from build123d import *

# Parameters (mm, degrees)
RESSALTO_EXTRUS_O1_DEPTH = 2
ESBO_O2_R                = 1.65
ESBO_O2_R_2              = 1.5
ESBO_O2_R_3              = 1
CORTE_EXTRUS_O1_DEPTH    = 3.0000001


with BuildPart() as part:
    # Esboço1 → Ressalto-extrusão1 (new body)
    with BuildSketch(Plane(origin=(0, 0, 0), x_dir=(1, 0, 0), z_dir=(0, 1, 0))):
        with BuildLine():
            Line((-57, 14.836150135), (-51, 9.5))
            Line((-51, 9.5), (-22.083647797, 9.5))
            add(Edge.make_bspline(
                [(22.083647797, 9.5), (0, 38), (-22.083647797, 9.5)],
                knots=[0.523598776, 0.523598776, 0.523598776, 2.617993878, 2.617993878, 2.617993878], degree=2, weights=[1, 0.5, 1]))
            Line((22.083647797, 9.5), (51, 9.5))
            Line((51, 9.5), (57, 14.836150135))
            Line((57, 14.836150135), (68, 14.836150135))
            Line((68, 14.836150135), (68, 8.836150135))
            Line((68, 8.836150135), (70.5, 8.836150135))
            Line((70.5, 8.836150135), (70.5, -7.163849865))
            Line((70.5, -7.163849865), (68, -7.163849865))
            Line((68, -7.163849865), (68, -13.163849865))
            Line((68, -13.163849865), (57, -13.163849865))
            Line((57, -13.163849865), (51, -9.5))
            Line((51, -9.5), (22.083647797, -9.5))
            add(Edge.make_bspline(
                [(-22.083647797, -9.5), (0, -38), (22.083647797, -9.5)],
                knots=[3.665191429, 3.665191429, 3.665191429, 5.759586532, 5.759586532, 5.759586532], degree=2, weights=[1, 0.5, 1]))
            Line((-22.083647797, -9.5), (-51, -9.5))
            Line((-51, -9.5), (-57, -13.163849865))
            Line((-57, -13.163849865), (-68, -13.163849865))
            Line((-68, -13.163849865), (-68, -7.163849865))
            Line((-68, -7.163849865), (-70.5, -7.163849865))
            Line((-70.5, -7.163849865), (-70.5, 8.836150135))
            Line((-70.5, 8.836150135), (-68, 8.836150135))
            Line((-68, 8.836150135), (-68, 14.836150135))
            Line((-68, 14.836150135), (-57, 14.836150135))
        make_face()
    extrude(amount=RESSALTO_EXTRUS_O1_DEPTH)

    # Esboço2 → Corte-extrusão1 (cut, through all)
    with BuildSketch(Plane(origin=(0, 2, 0), x_dir=(1, 0, 0), z_dir=(0, 1, 0))):
        with Locations((0, 15)):
            Circle(ESBO_O2_R)
        with Locations((10, 10.4)):
            Circle(ESBO_O2_R_2)
        with Locations((-10, 10.4)):
            Circle(ESBO_O2_R_2)
        with Locations((0, -15)):
            Circle(ESBO_O2_R)
        with Locations((10, -10.4)):
            Circle(ESBO_O2_R_2)
        with Locations((-10, -10.4)):
            Circle(ESBO_O2_R_2)
        with Locations((-9.5, 0)):
            Circle(ESBO_O2_R_3)
        with Locations((18.5, 0)):
            Circle(ESBO_O2_R_3)
        with BuildLine():
            Line((25.5, 3.836150135), (61.5, 3.836150135))
            ThreePointArc((61.5, 3.836150135), (62.207106781, 3.543256916), (62.5, 2.836150135))
            Line((62.5, 2.836150135), (62.5, -1.163849865))
            ThreePointArc((62.5, -1.163849865), (62.207106781, -1.870956646), (61.5, -2.163849865))
            Line((61.5, -2.163849865), (25.5, -2.163849865))
            ThreePointArc((25.5, -2.163849865), (24.792893219, -1.870956646), (24.5, -1.163849865))
            Line((24.5, -1.163849865), (24.5, 2.836150135))
            ThreePointArc((24.5, 2.836150135), (24.792893219, 3.543256916), (25.5, 3.836150135))
        make_face()
        with BuildLine():
            Line((-61.5, 3.836150135), (-25.5, 3.836150135))
            ThreePointArc((-25.5, 3.836150135), (-24.792893219, 3.543256916), (-24.5, 2.836150135))
            Line((-24.5, 2.836150135), (-24.5, -1.163849865))
            ThreePointArc((-24.5, -1.163849865), (-24.792893219, -1.870956646), (-25.5, -2.163849865))
            Line((-25.5, -2.163849865), (-61.5, -2.163849865))
            ThreePointArc((-61.5, -2.163849865), (-62.207106781, -1.870956646), (-62.5, -1.163849865))
            Line((-62.5, -1.163849865), (-62.5, 2.836150135))
            ThreePointArc((-62.5, 2.836150135), (-62.207106781, 3.543256916), (-61.5, 3.836150135))
        make_face()
        with BuildLine():
            Line((-6.5, 7), (15.5, 7))
            ThreePointArc((15.5, 7), (16.207106781, 6.707106781), (16.5, 6))
            Line((16.5, 6), (16.5, -6))
            ThreePointArc((16.5, -6), (16.207106781, -6.707106781), (15.5, -7))
            Line((15.5, -7), (-6.5, -7))
            ThreePointArc((-6.5, -7), (-7.207106781, -6.707106781), (-7.5, -6))
            Line((-7.5, -6), (-7.5, 6))
            ThreePointArc((-7.5, 6), (-7.207106781, 6.707106781), (-6.5, 7))
        make_face()
    extrude(amount=-CORTE_EXTRUS_O1_DEPTH, mode=Mode.SUBTRACT)


solid = part.part
Build history of the part. All positions in model axes, mm. A direction names the side the tool comes from. Give positions to 0.01 mm unless a question says otherwise; leave off trailing zeros. Write each loop counter-clockwise with the first axis right and the second up, starting at its lowest first coordinate (ties: lowest second). Pieces come first, ordered by that corner, then holes. Notation, with made-up numbers: (9.25, 33) - (23.25, 33) arc R28 ccw to (23.25, 67) - close; hole circle Ø9 at (-6, 78.25). An arc over 180 degrees is marked (long way). Use one line per item in the form item = value. Start each with the question number.
1. Probe line 1 (X direction, y = 1, z = 0); line 2 (Z direction, x = 38, y = 0.8); line 3 (X direction, y = 1.2, z = 10). List the from-to ranges inside material, lowest first. Write a range as [from, to].
2. Band-saw the part on B-B on y = 0.7. Count the separate pieces of the cut face and the enclosed holes in it, plus the area to 3 significant figures.
3. 3-axis set-ups, long thin cutter, end or side, ignore diameter. For faces 3 (the face through (0, 0, -9)), 4 (the face through (53.96, 0.99, -12.13)), 5 (the face through (54.042, 0.986, 11.358)): which of +Z, -Z, +X, -X, +Y, -Y reach the whole face in a straight line?
4. Band-saw the part on A-A on x = -31.5. Write the cut outline in (y, z), plus the area to 3 significant figures.
5. Two-plate mould, pull along X, no slides. Class faces 1 (the face through (-54.042, 0.986, -12.205)), 2 (the face through (0, 2, -9)): released by +X, released by -X, zero draft, split by the parting line, or undercut.
6. Drop flat-ended pins along their axis: pin 1 Ø0.6 at (x, y) = (41, 1) entering from +Z; pin 2 Ø0.6 at (x, y) = (6.5, 0.5) entering from +Z; pin 3 Ø1 at (x, y) = (-51, 0.5) entering from +Z. Give the stop position or say it passes through.
Conclusion:
q1.line_1 = [-70.5, -62.5], [-24.5, -10.5], [-8.5, -7.5], [16.5, 17.5], [19.5, 24.5], [62.5, 70.5]
q1.line_2 = [-9.5, -3.84], [2.16, 9.5]
q1.line_3 = [-68, -51.82], [-21.68, -11.45], [-8.55, 8.55], [11.45, 21.68], [51.82, 68]
q2.separate_pieces = 1
q2.enclosed_holes = 11
q2.area = 2,670 mm²
q3.face_3 = +Z, -Z, +X, -X, -Y
q3.face_4 = -Z, +Y, -Y
q3.face_5 = +Z, +Y, -Y
q4.outline = (0, -9.5) - (2, -9.5) - (2, -3.84) - (0, -3.84) - close; (0, 2.16) - (2, 2.16) - (2, 9.5) - (0, 9.5) - close
q4.area = 26.0 mm²
q5.face_1 = undercut
q5.face_2 = zero draft
q6.pin_1 = 9.5
q6.pin_2 = 18.43
q6.pin_3 = 9.81
